from build123d import *

# Parameters (mm, degrees)
SKETCH1_W           = 37
SKETCH1_H           = 55
SKETCH1_W_2         = 17
SKETCH1_H_2         = 3
BOSS_EXTRUDE1_DEPTH = 3
SKETCH2_W           = 37
SKETCH2_H           = 20
SKETCH2_R           = 3.175
BOSS_EXTRUDE2_DEPTH = 5
SKETCH3_W           = 37
SKETCH3_H           = 55
SKETCH3_W_2         = 17
SKETCH3_H_2         = 5
BOSS_EXTRUDE3_DEPTH = 2


with BuildPart() as part:
    # Sketch1 → Boss-Extrude1 (new body)
    with BuildSketch(Plane(origin=(0, 0, 0), x_dir=(1, 0, 0), z_dir=(0, 1, 0))):
        with Locations((18.5, -27.5)):
            Rectangle(SKETCH1_W, SKETCH1_H)
        with Locations((18.5, -5.5)):
            Rectangle(SKETCH1_W_2, SKETCH1_H_2, mode=Mode.SUBTRACT)
    extrude(amount=BOSS_EXTRUDE1_DEPTH)

    # Sketch2 → Boss-Extrude2 (add)
    with BuildSketch(Plane.XY.offset(55)):
        with Locations((18.5, 10)):
            Rectangle(SKETCH2_W, SKETCH2_H)
        with Locations((5, 13)):
            Circle(SKETCH2_R, mode=Mode.SUBTRACT)
        with Locations((30, 13)):
            Circle(SKETCH2_R, mode=Mode.SUBTRACT)
    extrude(amount=BOSS_EXTRUDE2_DEPTH)

    # Sketch3 → Boss-Extrude3 (add)
    with BuildSketch(Plane(origin=(0, 3, 0), x_dir=(1, 0, 0), z_dir=(0, 1, 0))):
        with Locations((18.5, -27.5)):
            Rectangle(SKETCH3_W, SKETCH3_H)
        with Locations((18.5, -5.5)):
            Rectangle(SKETCH3_W_2, SKETCH3_H_2, mode=Mode.SUBTRACT)
    extrude(amount=BOSS_EXTRUDE3_DEPTH)


solid = part.part
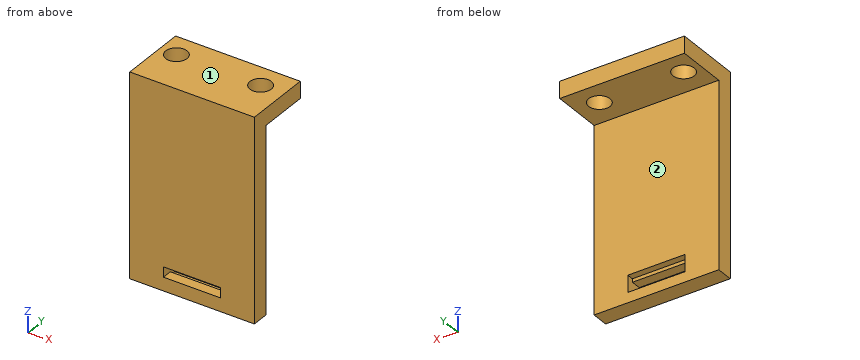
Geometry: final body of the model. Coordinates: model frame, mm. Face numbers are marked on the shaded views. A direction names the side the tool comes from. Give positions to 0.01 mm unless a question says otherwise; leave off trailing zeros. Order: outer loops, then holes, each group sorted by start corner. A loop starts at its lowest first (then second) coordinate and runs counter-clockwise, first axis right, second up. Notation, with made-up numbers: (11, 58) -> (27, 58) arc R22 cw to (27, 88) -> close; hole circle Ø7 at (-13, -40). An arc over 180 degrees is marked (long way). Answer as a JSON object with one key per item and string values.
Q1. Section C-C (x = 16.5). Output: boundary loops of the cut face in (y, z), plus the area to 3 significant figures.
Entries:
{"outline": "(0, 0) -> (5, 0) -> (5, 3) -> (3, 3) -> (3, 4) -> (0, 4) -> close; (0, 7) -> (3, 7) -> (3, 8) -> (5, 8) -> (5, 55) -> (20, 55) -> (20, 60) -> (0, 60) -> close", "area": "356 mm^2"}
Q2. Section A-A (x = 30). Output: boundary loops of the cut face in (y, z) (3 decimals), plus the area to 3 significant figures.
Entries:
{"outline": "(0, 0) -> (5, 0) -> (5, 55) -> (9.825, 55) -> (9.825, 60) -> (0, 60) -> close; (16.175, 55) -> (20, 55) -> (20, 60) -> (16.175, 60) -> close", "area": "343 mm^2"}
Q3. First-contact query: pin 1 (4 mm diameter, centred on y = 1.5, z = 6, fed in from -X); pin 2 (4 mm diameter, centred on x = 22.5, z = 25.5, fed in from +Y); pin 3 (0.8 mm diameter, centred on x = 18.5, z = 3.5, fed in from +Y). Flat tips, straight axial feed; report the tip coordinate or a pass-through.
Entries:
{"pin 1": "stops at x = 0", "pin 2": "stops at y = 5", "pin 3": "stops at y = 3"}
Q4. Section D-D (z = 39). Output: boundary loops of the cut face in (x, y), plus the area to 3 significant figures.
Entries:
{"outline": "(0, 0) -> (37, 0) -> (37, 5) -> (0, 5) -> close", "area": "185 mm^2"}
Q5. Section B-B (y = 13). Output: boundary loops of the cut face in (x, z) (3 decimals), plus the area to 4 significant figures.
Entries:
{"outline": "(0, 55) -> (1.825, 55) -> (1.825, 60) -> (0, 60) -> close; (8.175, 55) -> (26.825, 55) -> (26.825, 60) -> (8.175, 60) -> close; (33.175, 55) -> (37, 55) -> (37, 60) -> (33.175, 60) -> close", "area": "121.5 mm^2"}
Q6. Access query for the marked faces 1 and 2. Directions: +Z, -Z, +X, -X, +Y, -Y. A direction counts if a zero-diameter tool reaches every point of the face in a straight line with its end or side. Return the directions, or none.
Entries:
{"face 1": "+Z, +X, -X, +Y, -Y", "face 2": "-Z, +X, -X, +Y"}
Q7. Material intervals for probe 1 along Y at (x, z) = (5, 58.95) (3 decimals); probe 2 along Z at (x, y) = (16, 4.5); probe 3 along Y at (x, z) = (33, 5), sorted ascending.
Entries:
{"probe 1": "y = 0 to 9.825, 16.175 to 20", "probe 2": "z = 0 to 3, 8 to 60", "probe 3": "y = 0 to 5"}
